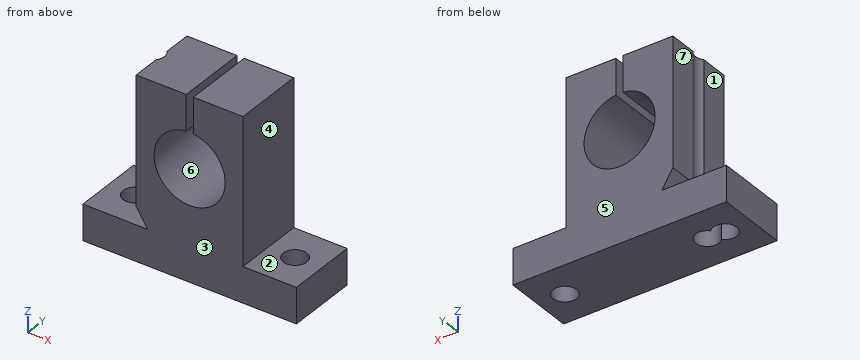
```python
from build123d import *

# Parameters (mm, degrees)
F1_DEPTH = 20
F3_D     = 6.6
F4_D     = 6.6
F5_D     = 6.6


with BuildPart() as f1:
    # F0 (on Front) → F1 (new body)
    with BuildSketch(Plane.XZ):
        with BuildLine():
            Line((-30, -25.5), (30, -25.5))
            Line((30, -25.5), (30, -15.5))
            Line((30, -15.5), (15, -15.5))
            Line((15, -15.5), (15, 25.5))
            Line((15, 25.5), (1.057532, 25.5))
            Line((1.057532, 25.5), (1.057532, 15.443924))
            ThreePointArc((1.057532, 15.443924), (-0.053951, -4.499854), (-0.950175, 15.454756))
            Line((-0.950175, 15.454756), (-0.950175, 25.5))
            Line((-0.950175, 25.5), (-15, 25.5))
            Line((-15, 25.5), (-15, -10.487244))
            Line((-15, -10.487244), (-11.823214, -15.5))
            Line((-11.823214, -15.5), (-15, -15.5))
            Line((-15, -15.5), (-30, -15.5))
            Line((-30, -15.5), (-30, -25.5))
        make_face()
    extrude(amount=F1_DEPTH)

    # F3 (through all)
    with Locations(Plane(origin=(0, 0, -25.5), x_dir=(1, 0, 0), z_dir=(0, 0, -1))):
        with Locations((-22.5, 10)):
            Hole(F3_D / 2)

    # F4 (through all)
    with Locations(Plane(origin=(0, 0, -25.5), x_dir=(1, 0, 0), z_dir=(0, 0, -1))):
        with Locations((22.5, 10)):
            Hole(F4_D / 2)

    # F5 (through all)
    with Locations(Plane(origin=(0, 0, -25.5), x_dir=(1, 0, 0), z_dir=(0, 0, -1))):
        with Locations((-17.5, 10)):
            Hole(F5_D / 2)


solid = f1.part
```
Model file for the job. Use its own axes, mm. Face numbers are marked on the shaded views. A direction names the side the tool comes from. Coordinates: 2 decimals unless noted, no trailing zeros. Order: outer loops, then holes, each group sorted by start corner. A loop starts at its lowest first (then second) coordinate and runs counter-clockwise, first axis right, second up. Notation, with made-up numbers: (-1, -19) -> (58, -19) arc R18 ccw to (58, -1) -> close; hole circle Ø9 at (29, 18.5). An arc over 180 degrees is marked (long way). Answer as a JSON object with one key per item and string values. Group by question number.
1) Cut at B-B, the plane x = -17.5. Write the cut outline in (y, z), then the cut area to 3 significant figures.
2) Cut at D-D, the plane z = 5.5. Write the cut outline in (x, y), then the cut area to 3 significant figures.
3) Flat gauge pins, fed straight in: pin 1 (4 mm diameter, centred on y = -10, z = 2.5, fed in from +X); pin 2 (4 mm diameter, centred on y = -3.5, z = -6.5, fed in from -X); pin 3 (12 mm diameter, centred on x = 24, y = -7.5, fed in from +Z). Where does each tip first touch, or does it go through?
4) Cut at C-C, the plane y = -10. Write the cut outline in (x, z).
5) Which spindle directions (+Z, -Z, +X, -X, +Y, -Y) get a long thin tool onto all of the face, cutting with end or side? Do the marked faces 1, 2 and 3. Say none if no direction does.
6) Pull direction X, two halves, no side cores. Call the marked faces 4, 5, 6 and 7: +X half, -X half, draft (parallel to the pull), parting line (faces both ways), or undercut.
7) Drill centre lines: L1, parallel to X at y = -10, z = -18.25; L2, parallel to X at y = -12.75, z = 5.5; L3, parallel to Y at x = -17.5, z = -19.75. Where is each one in solid material? Low to high.
8) Cut at A-A, the plane z = -17. Write the cut outline in (x, y), then the cut area to 3 significant figures.
Check values:
{
 "1": {"outline": "(-20, -25.5) -> (-13.3, -25.5) -> (-13.3, -15.5) -> (-20, -15.5) -> close; (-6.7, -25.5) -> (0, -25.5) -> (0, -15.5) -> (-6.7, -15.5) -> close", "area": "134 mm²"},
 "2": {"outline": "(-15, -20) -> (-10, -20) -> (-10, 0) -> (-15, 0) -> (-15, -7.85) arc R3.3 cw to (-15, -12.15) -> close; (10, -20) -> (15, -20) -> (15, 0) -> (10, 0) -> close", "area": "198 mm²"},
 "3": {"pin 1": "stops at x = 15", "pin 2": "stops at x = -15", "pin 3": "stops at z = -15.5"},
 "4": {"outline": "(-30, -25.5) -> (-25.8, -25.5) -> (-25.8, -15.5) -> (-30, -15.5) -> close; (-14.2, -25.5) -> (19.2, -25.5) -> (19.2, -15.5) -> (15, -15.5) -> (15, 25.5) -> (1.06, 25.5) -> (1.06, 15.44) arc R10 cw (long way) to (-0.95, 15.45) -> (-0.95, 25.5) -> (-14.2, 25.5) -> (-14.2, -11.75) -> (-11.82, -15.5) -> (-14.2, -15.5) -> close; (25.8, -25.5) -> (30, -25.5) -> (30, -15.5) -> (25.8, -15.5) -> close"},
 "5": {"face 1": "+Z, -X, +Y, -Y", "face 2": "+Z, +X, +Y, -Y", "face 3": "+Z, -Z, +X, -X, -Y"},
 "6": {"face 4": "+X half", "face 5": "draft", "face 6": "undercut", "face 7": "-X half"},
 "7": {"L1": "x = -30 to -25.8, -14.2 to 19.2, 25.8 to 30", "L2": "x = -15 to -10, 10 to 15", "L3": "y = -20 to -13.3, -6.7 to 0"},
 "8": {"outline": "(-30, -20) -> (30, -20) -> (30, 0) -> (-30, 0) -> close; hole (-20, -12.15) arc R3.3 ccw (long way) to (-20, -7.85) arc R3.3 ccw (long way) to start; hole circle Ø6.6 at (22.5, -10)", "area": "1,100 mm²"}
}
